Print and shaded views of the part. All mm, measured from the part's lowest x, y and z. A direction names the side the tool comes from. Coordinates: 2 decimals unless noted, no trailing zeros. Write each loop counter-clockwise with the first axis right and the second up, starting at its lowest first coordinate (ties: lowest second). Pieces come first, ordered by that corner, then holes. Notation, with made-up numbers: (-25, -7.5) -> (-15, -7.5) arc R34 ccw to (-15, 22.5) -> close; hole circle Ø6 at (71, 20). An arc over 180 degrees is marked (long way). Write item = value, one per line.
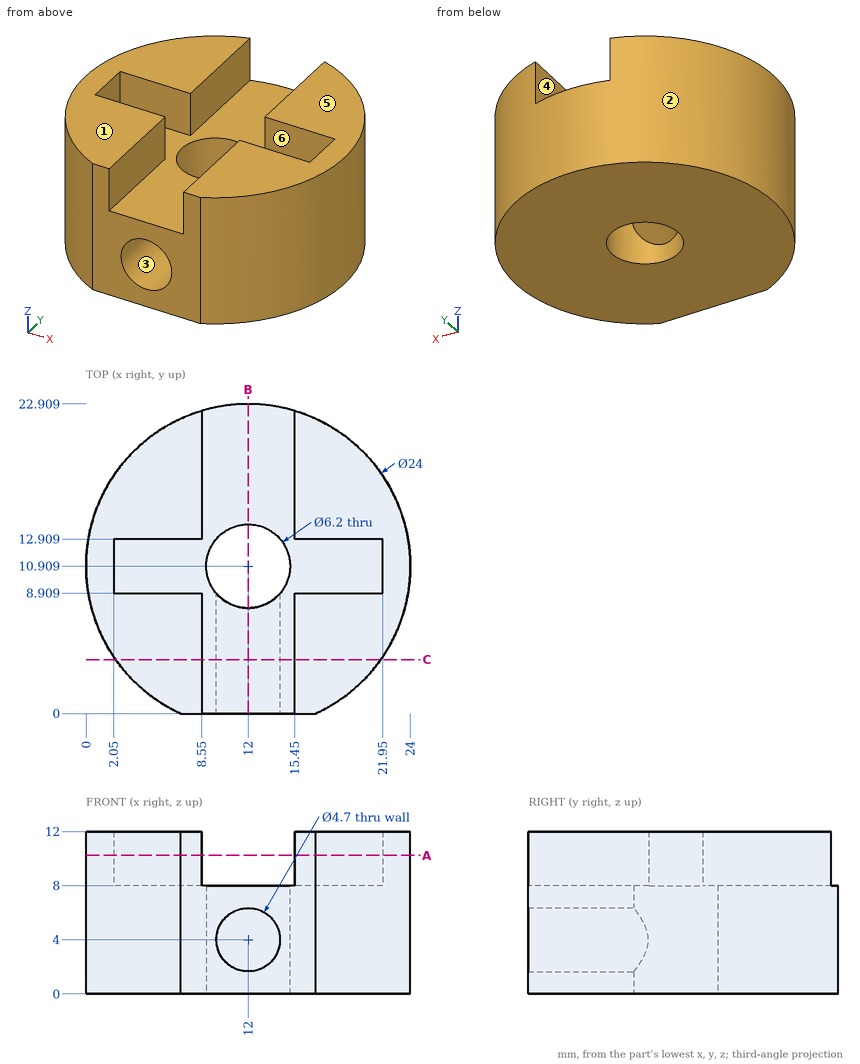
Q1. Which spindle directions (+Z, -Z, +X, -X, +Y, -Y) get a long thin tool onto all of the face, cutting with end or side? Do the marked faces 4, 5 and 6. Say none if no direction does.
Model answer:
face_4 = +Z, +Y, -Y
face_5 = +Z, +X, -X, +Y, -Y
face_6 = +Z
Q2. Saw through at C-C on y = 4. Give the cut face in (x, z).
Model answer:
outline = (2.19, 0) -> (21.81, 0) -> (21.81, 12) -> (15.45, 12) -> (15.45, 8) -> (8.55, 8) -> (8.55, 12) -> (2.19, 12) -> close; hole circle Ø4.7 at (12, 4)
Q3. Pin check, flat tips, straight feed: pin 1 (1.2 mm diameter, centred on x = 19, z = 10, fed in from +Y); pin 2 (6 mm diameter, centred on y = 17, z = 5.5, fed in from -X) (1 decimal); pin 3 (2 mm diameter, centred on y = 5.5, z = 10, fed in from -X); pin 4 (5.5 mm diameter, centred on x = 12, y = 10.91, fed in from -Z). Stop position of each tip, or through.
Model answer:
pin_1 = 21.06
pin_2 = 0.4
pin_3 = 0.84
pin_4 = through
Q4. Saw through at A-A on z = 10.25. Give the cut face in (x, y), and give its area (3 significant figures).
Model answer:
outline = (2.05, 8.91) -> (2.05, 12.91) -> (8.55, 12.91) -> (8.55, 22.4) arc R12 ccw to (7, 0) -> (8.55, 0) -> (8.55, 8.91) -> close; (15.45, 0) -> (17, 0) arc R12 ccw to (15.45, 22.4) -> (15.45, 12.91) -> (21.95, 12.91) -> (21.95, 8.91) -> (15.45, 8.91) -> close
area = 236 mm²
Q5. Probe line 1 (Z direction, x = 12, y = 6.5); line 2 (Y direction, x = 12, z = 6.5); line 3 (Y direction, x = 12, z = 6.25). List the from-to ranges inside material, lowest first. Write a range as from..to.
Model answer:
line_1 = 0..1.65, 6.35..8
line_2 = 0..7.81, 14.01..22.91
line_3 = 14.01..22.91
Q6. Mould opens along X. For the marked faces 1, 2 and 3 say: released by +X, released by -X, zero draft, split by the parting line, or undercut.
Model answer:
face_1 = zero draft
face_2 = split by the parting line
face_3 = undercut
Q7. Saw through at B-B on x = 12. Give the cut face in (y, z).
Model answer:
outline = (0, 0) -> (7.81, 0) -> (7.81, 1.65) -> (0, 1.65) -> close; (0, 6.35) -> (7.81, 6.35) -> (7.81, 8) -> (0, 8) -> close; (14.01, 0) -> (22.91, 0) -> (22.91, 8) -> (14.01, 8) -> close
